Drawing for the job (mm, zero at the part's lowest x, y, z). A direction names the side the tool comes from. Round coordinates to 2 decimals unless told otherwise and drop trailing zeros. Order: outer loops, then holes, each group sorted by start corner. A loop starts at its lowest first (then second) coordinate and runs counter-clockwise, first axis right, second up. Notation, with made-up numbers: M 29,56 L 65,56 A15 ccw 65,66 Z; hole C 27.5,56 d6. An arc over 180 degrees is marked long. One line per item, written item: value. Start each with the question number.
Item 1: Band-saw the part on C-C, the plane y = 3. Write the cut outline in (x, z), then the cut area to 3 significant figures.
Item 2: Probe L1, parallel to Y at x = 11, z = 11.2; L2, parallel to Y at x = 3, z = 12; L3, parallel to X at y = 11.75, z = 11.75. List the from-to ranges inside material, lowest first.
Item 3: Tool access for the marked faces 5 and 6: list every direction of +Z, -Z, +X, -X, +Y, -Y with a clear straight run to the whole face (end or side of a thin tool).
Item 4: Band-saw the part on A-A, the plane x = 11. Write the cut outline in (y, z), then the cut area to 3 significant figures.
Item 5: Pin check, flat tips, straight feed: pin 1 (1 mm diameter, centred on y = 10, z = 6.5, fed in from -X); pin 2 (2 mm diameter, centred on x = 11, y = 19, fed in from +Z); pin 3 (8 mm diameter, centred on x = 4, z = 13.5, fed in from +Y); pin 4 (3 mm diameter, centred on y = 6.5, z = 11.5, fed in from -X). Stop position of each tip, or through.
Item 6: Two-plate mould, pull along X, no slides. Class the marked faces 1, 2, 3 and 4: +X half, -X half, draft (parallel to the pull), parting line (faces both ways), or undercut.
Item 7: Band-saw the part on D-D, the plane x = 8.75. Write the cut outline in (y, z), then the cut area to 3 significant figures.
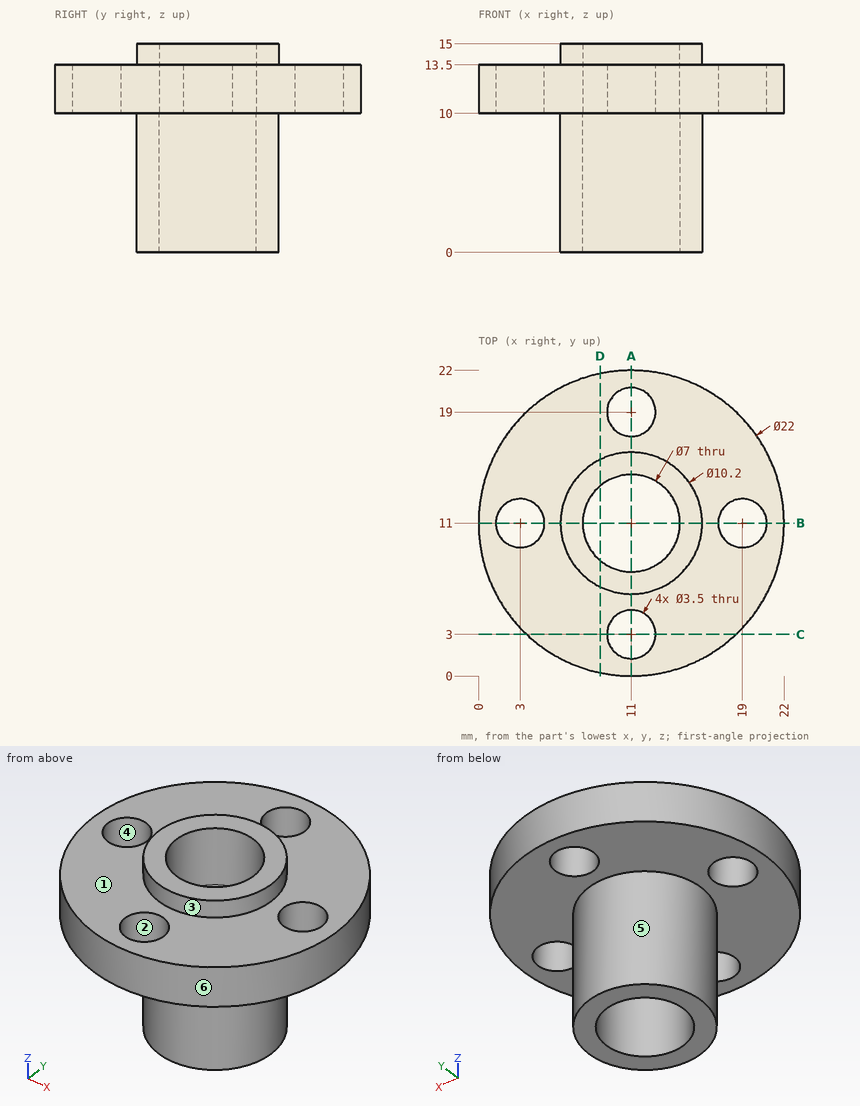
Output:
1. outline: M 3.45,10 L 9.25,10 L 9.25,13.5 L 3.45,13.5 Z; M 12.75,10 L 18.55,10 L 18.55,13.5 L 12.75,13.5 Z
1. area: 40.6 mm²
2. L1: y = 0 to 1.25, 4.75 to 7.5, 14.5 to 17.25, 20.75 to 22
2. L2: y = 3.45 to 9.25, 12.75 to 18.55
2. L3: x = 0.03 to 1.42, 4.58 to 7.58, 14.42 to 17.42, 20.58 to 21.97
3. face 5: -Z
3. face 6: +Z, -Z
4. outline: M 0,10 L 1.25,10 L 1.25,13.5 L 0,13.5 Z; M 4.75,10 L 5.9,10 L 5.9,0 L 7.5,0 L 7.5,15 L 5.9,15 L 5.9,13.5 L 4.75,13.5 Z; M 14.5,0 L 16.1,0 L 16.1,10 L 17.25,10 L 17.25,13.5 L 16.1,13.5 L 16.1,15 L 14.5,15 Z; M 20.75,10 L 22,10 L 22,13.5 L 20.75,13.5 Z
4. area: 64.8 mm²
5. pin 1: stops at x = 5.92
5. pin 2: passes through
5. pin 3: stops at y = 21.58
5. pin 4: stops at x = 0.42
6. face 1: draft
6. face 2: undercut
6. face 3: parting line
6. face 4: undercut
7. outline: M 0.23,10 L 6.42,10 L 6.42,0 L 8.32,0 L 8.32,15 L 6.42,15 L 6.42,13.5 L 0.23,13.5 Z; M 13.68,0 L 15.58,0 L 15.58,10 L 21.77,10 L 21.77,13.5 L 15.58,13.5 L 15.58,15 L 13.68,15 Z
7. area: 100 mm²
